Check sheet for the modelled part. Datum: model origin and axes. Units: mm. A direction names the side the tool comes from. Give positions to 0.01 mm unless a question says otherwise; leave off trailing zeros. Order: outer loops, then holes, each group sorted by start corner. A loop starts at its lowest first (then second) coordinate and runs counter-clockwise, first axis right, second up.
Item 1: Material ranges on line 1 along X through (y, z) = (4.25, 21.35); line 2 along Y through (x, z) = (-3.5, 22); line 3 along X through (y, z) = (-4, 22.25), recorded low to high.
Item 2: Release check for a two-part mould opening along Y. For faces 3 (the cylindrical face through (-1.73, -7.81, 23.93)), 4 (the flat face through (-2, 2, 29)), 5 (the cylindrical face through (4.987, 3.574, 20.972)) record: released by +Y, released by -Y, zero draft, split by the parting line, or undercut.
Item 3: Gauge pin test, flat ends, axial feed: P1, Ø0.6, axis at x = -4, y = -4.5, coming from the -Z side; P2, Ø4, axis at y = -5, z = 28, coming from the -X side; P3, Ø4, axis at x = -4.5, z = 22, coming from the +Y side. Record the tip position at first contact, or that the pin passes through.
Item 4: Sectioned sample at A-A on x = 0. Record the boundary of the cut face in (y, z), and give its area (3 significant figures).
Item 5: Sectioned sample at C-C on z = 22.5. Record the boundary of the cut face in (x, y), and give its area (3 significant figures).
Item 6: Access from +Z, -Z, +X, -X, +Y, -Y to the whole of each face (thin tool, end or side, straight path). Record for faces 1 (the flat face through (-2, 2, 19)), 2 (the cylindrical face through (-3.574, 4.987, 20.972)).
Item 7: Sectioned sample at D-D on x = 3.5. Record the boundary of the cut face in (y, z).
from build123d import *

# Parameters (mm, degrees)
CYLINDER985_R     = 1
CYLINDER985_DEPTH = 20
CYLINDER982_R     = 1
CYLINDER982_DEPTH = 20
CYLINDER983_R     = 1
CYLINDER983_DEPTH = 20
CYLINDER984_R     = 1
CYLINDER984_DEPTH = 20
TUBE080_R         = 8
TUBE080_R_2       = 2.6
TUBE080_DEPTH     = 10


with BuildPart() as obj1:
    # Cylinder985 → Cylinder985 (new body)
    with BuildSketch(Plane(origin=(4.25, -4.25, -88), x_dir=(0, 1, 0), z_dir=(0, 0, 1))):
        Circle(CYLINDER985_R)
    extrude(amount=CYLINDER985_DEPTH)


with BuildPart() as obj2:
    # Cylinder982 → Cylinder982 (new body)
    with BuildSketch(Plane(origin=(4.25, 4.25, -88), x_dir=(-1, 0, 0), z_dir=(0, 0, 1))):
        Circle(CYLINDER982_R)
    extrude(amount=CYLINDER982_DEPTH)


with BuildPart() as obj3:
    # Cylinder983 → Cylinder983 (new body)
    with BuildSketch(Plane(origin=(-4.25, 4.25, -88), x_dir=(0, -1, 0), z_dir=(0, 0, 1))):
        Circle(CYLINDER983_R)
    extrude(amount=CYLINDER983_DEPTH)


with BuildPart() as compound810:
    # Cylinder984 → Cylinder984 (new body)
    with BuildSketch(Plane(origin=(-4.25, -4.25, -88), x_dir=(1, 0, 0), z_dir=(0, 0, 1))):
        Circle(CYLINDER984_R)
    extrude(amount=CYLINDER984_DEPTH)

    # Compound810: union obj1, obj2, obj3
    add(obj1.part)
    add(obj2.part)
    add(obj3.part)


with BuildPart() as compound810_1:
    # Compound810 placement: moved
    add(compound810.part.moved(Location((0, 0, 91))))


with BuildPart() as cut091:
    # Tube080 → Tube080 (new body)
    with BuildSketch(Plane.XY.offset(19)):
        Circle(TUBE080_R)
        Circle(TUBE080_R_2, mode=Mode.SUBTRACT)
    extrude(amount=TUBE080_DEPTH)

    # Cut091: cut Compound810
    add(compound810_1.part, mode=Mode.SUBTRACT)


solid = cut091.part
Report:
1. line 1: x = -6.78 to -5.25, -3.25 to 3.25, 5.25 to 6.78
1. line 2: y = -7.19 to -4.91, -3.59 to 3.59, 4.91 to 7.19
1. line 3: x = -6.93 to -5.22, -3.28 to 3.28, 5.22 to 6.93
2. face 3: split by the parting line
2. face 4: zero draft
2. face 5: undercut
3. P1: stops at z = 23
3. P2: stops at x = -7.42
3. P3: stops at y = 7.6
4. outline: (-8, 19) - (-2.6, 19) - (-2.6, 29) - (-8, 29) - close; (2.6, 19) - (8, 19) - (8, 29) - (2.6, 29) - close
4. area: 108 mm2
5. outline: circle Ø16 at (0, 0); hole circle Ø2 at (-4.25, -4.25); hole circle Ø2 at (-4.25, 4.25); hole circle Ø5.2 at (0, 0); hole circle Ø2 at (4.25, -4.25); hole circle Ø2 at (4.25, 4.25)
5. area: 167 mm2
6. face 1: -Z, +X, -X, +Y, -Y
6. face 2: -Z
7. outline: (-7.19, 19) - (-4.91, 19) - (-4.91, 23) - (-3.59, 23) - (-3.59, 19) - (3.59, 19) - (3.59, 23) - (4.91, 23) - (4.91, 19) - (7.19, 19) - (7.19, 29) - (-7.19, 29) - close
